Autodesk Inventor part; units mm, degrees
ref_plane "YZ Plane" through (0, 0, 0) normal (1, 0, 0) x (0, 1, 0)
ref_plane "XZ Plane" through (0, 0, 0) normal (0, 1, 0) x (-1, 0, 0)
ref_plane "XY Plane" through (0, 0, 0) normal (0, 0, 1) x (1, 0, 0)
sketch "Эскиз1" plane through (0, 0, 0) normal (1, 0, 0) x (0, 1, 0)
  line L0 (0, 2.8) -> (29, 2.8)
  line L1 (0, 6) -> (15, 6)
  line L2 (15, 6) -> (15, 5)
  line L3 (22, 5) -> (22, 6)
  line L4 (22, 6) -> (29, 6)
  line L5 (29, 6) -> (29, 2.8)
  line L6 (22, 5) -> (15, 5)
  line L7 (0, 6) -> (0, 2.8)
  line L8 (32.1482, 0) -> (-3.0834, 0)
  point P0 (0, 0)
revolve "Вращение1" add sketch "Эскиз1" angle 360 about axis through (0, 32.1482, 0) along (0, -1, 0)
chamfer "Фаска1" distance 1 angle 45 2 edges at (0, 15, -6) (0, 22, -6)
chamfer "Фаска2" distance 0.4 angle 45 4 edges at (0, 29, -2.8) (0, 29, -6) (0, 0, -6) (0, 0, -2.8)
properties part number "prostavka"
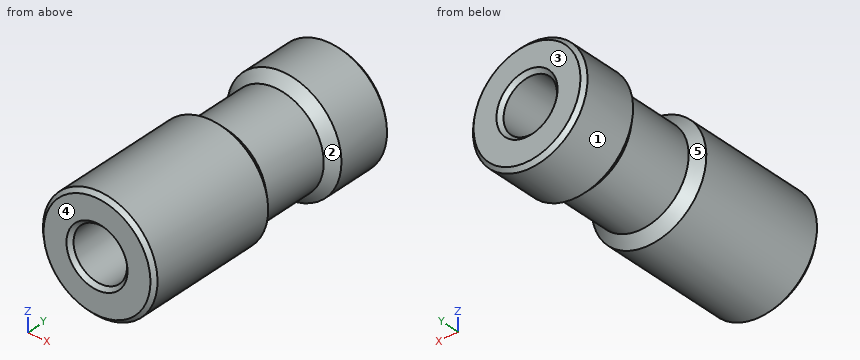
Geometry check sheet. Reference: the model listing, model coordinates, mm. Face numbers are marked on the shaded views. A direction names the side the tool comes from. Coordinates: 2 decimals unless noted, no trailing zeros. Order: outer loops, then holes, each group sorted by start corner. A loop starts at its lowest first (then second) coordinate and runs counter-clockwise, first axis right, second up. Notation, with made-up numbers: (50.5, 14) -> (87.5, 14) arc R18 ccw to (87.5, 30) -> close; hole circle Ø11 at (27.25, 69.5). An arc over 180 degrees is marked (long way). Use a Markdown table: item, result. Add a question column.
1. Material ranges on L1, parallel to X at y = 18, z = 0; L2, parallel to X at y = 7.5, z = 0, recorded low to high.
2. Go/stop test with flat-tipped pins: pin 1 Ø1 at (x, z) = (-1.5, 2) entering from -Y; pin 2 Ø1 at (x, y) = (-1.5, 4) entering from +Z. Record where each tip stops, or that it passes through.
3. Mould release check, pull along Y, two halves, no side actions. Record for the marked faces 1, 2 and 3: pulls with the +Y half, pulls with the -Y half, needs draft (parallel to the pull), parting line crosses it, or undercut.
4. Set-up check for the marked faces 4 and 5: record each of +Z, -Z, +X, -X, +Y, -Y from which the full face is reachable in a straight line by a thin tool's end or side.
5. Cross-section at C-C (y = 18). Enter the section's corners in (x, z), and give its area (3 significant figures).
Filled sheet:
| question | item | result |
|---|---|---|
| 1 | L1 | -5 to -2.8, 2.8 to 5 |
| 1 | L2 | -6 to -2.8, 2.8 to 6 |
| 2 | pin 1 | y = 0.2 |
| 2 | pin 2 | z = 5.92 |
| 3 | face 1 | needs draft |
| 3 | face 2 | undercut |
| 3 | face 3 | pulls with the +Y half |
| 4 | face 4 | +Z, -Z, +X, -X, -Y |
| 4 | face 5 | none |
| 5 | outline | circle Ø10 at (0, 0); hole circle Ø5.6 at (0, 0) |
| 5 | area | 53.9 mm2 |
